Autodesk Inventor part; units mm, degrees
ref_plane "YZ Plane" through (0, 0, 0) normal (1, 0, 0) x (0, 1, 0)
ref_plane "XZ Plane" through (0, 0, 0) normal (0, 1, 0) x (-1, 0, 0)
ref_plane "XY Plane" through (0, 0, 0) normal (0, 0, 1) x (1, 0, 0)
sketch "Sketch2" plane through (0, 0, 0) normal (0, 1, 0) x (-1, 0, 0)
  circle A0 centre (0, 0) radius 2.0955
  arc A1 (-4.7625, 0) -> (-4.7625, 0) centre (0, 0) ccw
  circle A2 centre (0.0001, -38.1) radius 2.0955
  arc A3 (-4.7625, -38.1) -> (4.7628, -38.1) centre (0.0001, -38.1) ccw
  line L0 (4.7625, 0) -> (4.7628, -38.1)
  line L1 (-4.7625, 0) -> (-4.7625, -38.1)
  arc A4 (4.7625, 0) -> (-4.7625, 0) centre (0, 0) ccw
  dimension "d0" = 4.191
  dimension "d1" = 2.667
  dimension "d2" = 4.191
  dimension "d5" = 38.1
extrude "Extrusion1" add sketch "Sketch2" along normal blind 1.5875
properties part number "straight_gusset" material "Acetal Resin, White"
Build history of the part. All positions in model axes, mm. Give positions to 0.01 mm unless a question says otherwise; leave off trailing zeros. Order: outer loops, then holes, each group sorted by start corner. A loop starts at its lowest first (then second) coordinate and runs counter-clockwise, first axis right, second up. Notation, with made-up numbers: M 31.5,79 L 36.5,79 A26 cw 36.5,106 Z; hole C 15,86 d1. An arc over 180 degrees is marked long. Write item = value, one per line. Start each with the question number.
(1) Slice it at C-C on z = 0.5. Write the cut outline in (x, y).
(2) Slice it at B-B on y = 0.55. Write the cut outline in (x, z) (1 decimal), plus the area to 3 significant figures.
(3) Slice it at A-A on x = 0. Write the cut outline in (y, z), plus the area to 3 significant figures.
(4) Slice it at D-D on x = 2.5. Write the cut outline in (y, z).
(5) Two-plate mould, pull along Z, no slides. Class faces 1 (the cylindrical face through (-2, 0.78, -0.63)), 2 (the cylindrical face through (0.1, 0.78, 4.76)), 3 (the cylindrical face through (0.454, 0.783, -36.054)), 4 (the flat face through (0, 1.588, -19)): released by +Z, released by -Z, zero draft, split by the parting line, or undercut.
(6) Probe L1, parallel to Z at x = 0, y = 0.65; L2, parallel to Z at x = -1.5, y = 0.5; L3, parallel to X at y = 0.6, z = -38. List the from-to ranges inside material, lowest first. Write a range as [from, to].
Responses:
q1.outline = M -4.74,0 L -2.03,0 L -2.03,1.59 L -4.74,1.59 Z; M 2.03,0 L 4.74,0 L 4.74,1.59 L 2.03,1.59 Z
q2.outline = M -4.8,-38.1 A4.8 ccw 4.8,-38.1 L 4.8,0 A4.8 ccw -4.8,0 Z; hole C 0,-38.1 d4.2; hole C 0,0 d4.2
q2.area = 407 mm2
q3.outline = M 0,-42.86 L 1.59,-42.86 L 1.59,-40.2 L 0,-40.2 Z; M 0,-36 L 1.59,-36 L 1.59,-2.1 L 0,-2.1 Z; M 0,2.1 L 1.59,2.1 L 1.59,4.76 L 0,4.76 Z
q3.area = 62.3 mm2
q4.outline = M 0,-42.15 L 1.59,-42.15 L 1.59,4.05 L 0,4.05 Z
q5.face_1 = undercut
q5.face_2 = released by +Z
q5.face_3 = undercut
q5.face_4 = zero draft
q6.L1 = [-42.86, -40.2], [-36, -2.1], [2.1, 4.76]
q6.L2 = [-42.62, -39.56], [-36.64, -1.46], [1.46, 4.52]
q6.L3 = [-4.76, -2.09], [2.09, 4.76]
